from build123d import *

# Parameters (mm, degrees)
F3_DEPTH = 0.2
F6_DEPTH = 0.2
F7_COUNT = 4


# Not quite as in the source:
# - a feature names something its author has since deleted; it is built from what else it names


with BuildPart() as f1:
    # F0 (on Front) → F1 (revolve)
    with BuildSketch(Plane.XZ):
        with BuildLine():
            Line((0, 19.7569444444), (0, 0))
            Line((0, 0), (0.4409722222, 0))
            Line((0.4409722222, 0), (0.4409722222, 19.0625))
            ThreePointArc((0.4409722222, 19.0625), (0.4053949582, 19.3321442616), (0.3010981711, 19.5833333333))
            ThreePointArc((0.3010981711, 19.5833333333), (0.1737821384, 19.7104325641), (0, 19.7569444444))
        make_face()
    revolve(axis=Axis((0, 0, 9.8784722222), (0, 0, 1)))

    # F2 (on Front) → F3 (join, symmetric)
    with BuildSketch(Plane.XZ):
        Polygon((0, 12.279863856), (0, 3.9918203777), (1.3194444444, 4.9305555556), (1.3194444444, 8.0555555556), align=None)
        Polygon((0, 2.1539925494), (0, 0), (0.4409722222, 0), (0.4409722222, -0.2083333333), (0.3715277778, -0.2083333333), (0.3715277778, -0.3819444444), (0.5902777778, -0.3819444444), (0.5902777778, 0.8333333333), (1.6319444444, 0.8333333333), (1.6319444444, 1.25), align=None)
    extrude(amount=F3_DEPTH, both=True)

    # F5 (on face) → F6 (join, symmetric)
    with BuildSketch(Plane(origin=(0, 0, 0), x_dir=(0.7071067812, -0.7071067812, 0), z_dir=(-0.7071067812, -0.7071067812, 0))):
        Polygon((0, 16.5328663793), (0.6423611111, 17.03125), (0.6423611111, 17.6909722222), (0, 18.1893558429), align=None)
    extrude(amount=F6_DEPTH, both=True)

    # F7: F1 ×4 about axis
    f7_axis = Axis((0, 0, 0), (0, 0, 1))


with BuildPart() as f1_1:
    add(f1.part)
    for i in range(1, F7_COUNT):
        add(f1.part.rotate(f7_axis, i * 360 / F7_COUNT))


solid = f1_1.part
Can you work these out from the model? Positions are in its coordinate system, mm. A direction names the side the tool comes from. Coordinates: 2 decimals unless noted, no trailing zeros. Loops run counter-clockwise (first coordinate to the right, second up) from the corner with the lowest first, then second, coordinate; pieces in that order, holes last. Notation, with made-up numbers: M 70,89 L 96,89 A18 ccw 96,115 Z; hole C 28.25,12.25 d8. An arc over 180 degrees is marked long. Return JSON: item names as keys, results as strings. Group by question number.
Item 1: Imagine slicing it at C-C (y = -0.9). Please give me the cut outline in (x, z), and give its area (3 significant figures).
Item 2: Imagine slicing it at B-B (x = 0.8). Please give me the cut outline in (y, z).
Item 3: I'm going to push flat-ended pins straight in: pin 1 Ø1 at (y, z) = (-1, 0.5) entering from +X; pin 2 Ø1 at (x, z) = (-1, 6.5) entering from -Y; pin 3 Ø1.4 at (x, z) = (1, 0.5) entering from +Y. Where does each tip first touch, or does it pass through?
Item 4: On a 3-axis mill with a long thin cutter (end or side, diameter ignored), from which of +Z, -Z, +X, -X, +Y, -Y can I reach the whole of each face in a straight line? I mean faces 3 (the flat face through (1, 0.2, 1)), 4 (the flat face through (0.2, -1, 1)), 5 (the flat face through (-0.2, -1, 7)), 6 (the flat face through (-0.2, 1, 7)), 7 (the cylindrical face through (-0.44, 0.02, 11.78)). Say none if no direction works.
Item 5: Imagine slicing it at D-D (z = 10.5). Please give me the cut outline in (x, y), and give its area (3 significant figures).
Item 6: Thinking about a two-plate mould opening in Z: for faces 1 (the flat face through (-1, 0.2, 1)), 2 (the flat face through (0, 0, 0)), which applies, released by +Z, released by -Z, zero draft, split by the parting line, or undercut?
Item 7: Imagine slicing it at A-A (z = 6.75). Please give me the cut outline in (x, y), and give its area (3 significant figures).
Item 8: If I drill on L1, parallel to X at y = 1.2, z = 1; L2, parallel to Y at x = -0.2, z = 14.25, over which ranges is the centre line in solid material (lowest first)? Write a range as from..to.
Verdict:
{
 "1": {"outline": "M -0.2,0.83 L 0.2,0.83 L 0.2,1.66 L -0.2,1.66 Z; M -0.2,4.63 L 0.2,4.63 L 0.2,9.4 L -0.2,9.4 Z", "area": "2.24 mm^2"},
 "2": {"outline": "M -0.2,0.83 L 0.2,0.83 L 0.2,1.71 L -0.2,1.71 Z; M -0.2,4.56 L 0.2,4.56 L 0.2,9.72 L -0.2,9.72 Z"},
 "3": {"pin 1": "stops at x = 0.2", "pin 2": "stops at y = -0.2", "pin 3": "stops at y = 0.32"},
 "4": {"face 3": "-Z, +X, +Y", "face 4": "-Z, +X, -Y", "face 5": "-Z, -X, -Y", "face 6": "-Z, -X, +Y", "face 7": "none"},
 "5": {"outline": "M -0.56,-0.2 L -0.39,-0.2 A0.44 ccw -0.2,-0.39 L -0.2,-0.56 L 0.2,-0.56 L 0.2,-0.39 A0.44 ccw 0.39,-0.2 L 0.56,-0.2 L 0.56,0.2 L 0.39,0.2 A0.44 ccw 0.2,0.39 L 0.2,0.56 L -0.2,0.56 L -0.2,0.39 A0.44 ccw -0.39,0.2 L -0.56,0.2 Z", "area": "0.820 mm^2"},
 "6": {"face 1": "zero draft", "face 2": "undercut"},
 "7": {"outline": "M -1.32,-0.2 L -0.39,-0.2 A0.44 ccw -0.2,-0.39 L -0.2,-1.32 L 0.2,-1.32 L 0.2,-0.39 A0.44 ccw 0.39,-0.2 L 1.32,-0.2 L 1.32,0.2 L 0.39,0.2 A0.44 ccw 0.2,0.39 L 0.2,1.32 L -0.2,1.32 L -0.2,0.39 A0.44 ccw -0.39,0.2 L -1.32,0.2 Z", "area": "2.04 mm^2"},
 "8": {"L1": "x = -0.2..0.2", "L2": "y = -0.39..0.39"}
}
